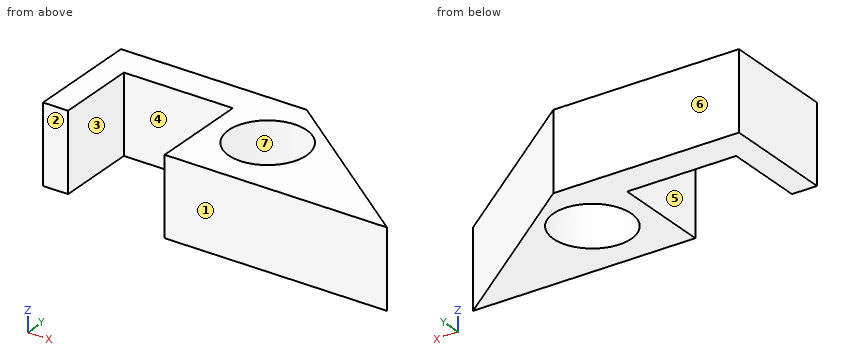
```python
from build123d import *

# Parameters (mm, degrees)
F0_R     = 6.35
F1_DEPTH = 12.7
F2_W     = 4.087012
F2_H     = 12.7
F3_DEPTH = 8.8138
F5_DEPTH = 12.701


with BuildPart() as f1:
    # F0 (on Top) → F1 (new body)
    with BuildSketch(Plane.XY):
        Polygon((-44.868298, 5.242039), (-44.868298, 0), (-44.868298, -4.353558), (-40.781286, -4.353558), (-40.781286, 0), (-23.011663, 0), (-23.011663, -16.081509), (13.23837, -16.081509), (13.23837, 5.242039), (-23.011663, 5.242039), (-40.781286, 5.242039), align=None)
        with Locations((-13.593762, -5.419735)):
            Circle(F0_R, mode=Mode.SUBTRACT)
    extrude(amount=F1_DEPTH)

    # F2 (on face) → F3 (join)
    with BuildSketch(Plane.XZ.offset(4.353558)):
        with Locations((-42.824792, 6.35)):
            Rectangle(F2_W, F2_H)
    extrude(amount=F3_DEPTH)

    # F4 (on face) → F5 (cut, through all)
    with BuildSketch(Plane(origin=(0, 0, 0), x_dir=(1, 0, 0), z_dir=(0, 0, -1))):
        Polygon((13.23837, -5.242039), (13.23837, 16.081509), (-14.590898, -5.242039), align=None)
    extrude(amount=-F5_DEPTH, mode=Mode.SUBTRACT)


solid = f1.part
```
The listing builds one solid part. Answer for the finished solid, in the listing's coordinates (mm). Face numbers are marked on the shaded views. A direction names the side the tool comes from. Coordinates: 2 decimals unless noted, no trailing zeros. Write each loop counter-clockwise with the first axis right and the second up, starting at its lowest first coordinate (ties: lowest second). Pieces come first, ordered by that corner, then holes. Notation, with made-up numbers: (77.5, 50) - (92.5, 50) arc R22 cw to (92.5, 61) - close; hole circle Ø3 at (4, -24.75). An arc over 180 degrees is marked (long way). One line per item, written item: value.
1) Find section A-A (x = -13.5). Give the vertices of the cut face in (y, z), and give its area (3 significant figures).
Geometry check:
outline: (-16.08, 0) - (-11.77, 0) - (-11.77, 12.7) - (-16.08, 12.7) - close; (0.93, 0) - (4.41, 0) - (4.41, 12.7) - (0.93, 12.7) - close
area: 98.9 mm2
2) Find section D-D (x = -28). Give the vertices of the cut face in (y, z).
Geometry check:
outline: (0, 0) - (5.24, 0) - (5.24, 12.7) - (0, 12.7) - close
3) For a pull along Y with two mould halves and no side action, classify the marked faces 4, 5, 6 and 7 as pulls with the +Y half, pulls with the -Y half, needs draft (parallel to the pull), parting line crosses it, or undercut.
Geometry check:
face 4: pulls with the -Y half
face 5: needs draft
face 6: pulls with the +Y half
face 7: undercut
4) Find section C-C (z = 4.75). Give the vertices of the cut face in (x, y), and give its area (3 significant figures).
Geometry check:
outline: (-44.87, -13.17) - (-40.78, -13.17) - (-40.78, 0) - (-23.01, 0) - (-23.01, -16.08) - (13.24, -16.08) - (-14.59, 5.24) - (-44.87, 5.24) - close; hole circle Ø12.7 at (-13.59, -5.42)
area: 518 mm2
5) A tool of negligible diameter and unlimited length cuts with its end or side. For the marked faces 1, 2 and 3, from which of +Z, -Z, +X, -X, +Y, -Y can it reach the whole face along a straight path? Write none if from no direction.
Geometry check:
face 1: +Z, -Z, +X, -X, -Y
face 2: +Z, -Z, -X, -Y
face 3: +Z, -Z, -Y
6) Each of these flat-tipped pins is pushed along its axis until it touches: pin 1 Ø1.2 at (x, z) = (-44, 6) entering from -Y; pin 2 Ø3 at (x, y) = (-38, -7) entering from +Z; pin 3 Ø4 at (y, z) = (1.5, 8.5) entering from +X; pin 4 Ø5 at (x, z) = (-28, 1.5) entering from -Y. Where does it stop, or does it pass through?
Geometry check:
pin 1: stops at y = -13.17
pin 2: passes through
pin 3: stops at x = -7.1
pin 4: stops at y = 0
7) Find section B-B (y = -2.25). Give the vertices of the cut face in (x, z).
Geometry check:
outline: (-44.87, 0) - (-40.78, 0) - (-40.78, 12.7) - (-44.87, 12.7) - close; (-23.01, 0) - (-19.1, 0) - (-19.1, 12.7) - (-23.01, 12.7) - close; (-8.09, 0) - (-4.81, 0) - (-4.81, 12.7) - (-8.09, 12.7) - close
8) Consider line 1 along X through (y, z) = (-6.25, 7.25); line 2 along X through (y, z) = (-4.75, 10.5); line 3 along Y through (x, z) = (-31.5, 12). Determine where each line is inside the solid, lowest interval first. Write a range as from..to.
Geometry check:
line 1: x = -44.87..-40.78, -23.01..-19.89, -7.3..0.41
line 2: x = -44.87..-40.78, -23.01..-19.91, -7.28..-1.55
line 3: y = 0..5.24
